Geometry check sheet. Reference: the model listing, model coordinates, mm. Give positions to 0.01 mm unless a question says otherwise; leave off trailing zeros. Write each loop counter-clockwise with the first axis right and the second up, starting at its lowest first coordinate (ties: lowest second). Pieces come first, ordered by that corner, then holes. Notation, with made-up numbers: (65, 21.5) - (123, 21.5) arc R13 ccw to (123, 42.5) - close; hole circle Ø10 at (-3.75, 77). An arc over 180 degrees is marked (long way). Use a Markdown table: item, result.
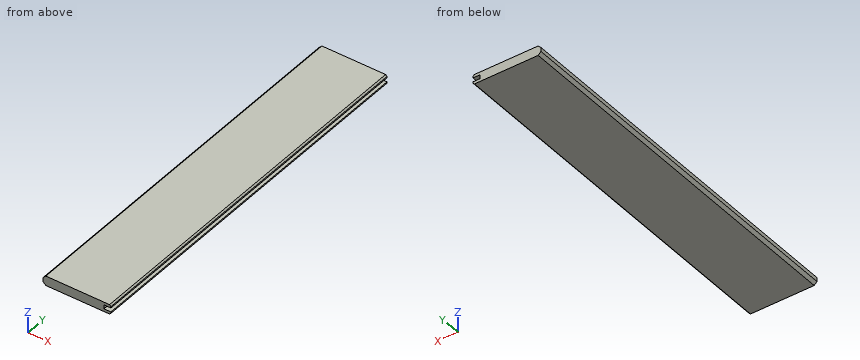
```python
from build123d import *

# Parameters (mm, degrees)
F1_DEPTH = 685.8
F2_SIZE  = 2.54
F3_SIZE  = 5.07999
F4_W     = 25.4
F4_H     = 7.3152
F5_DEPTH = 685.801


# Not quite as in the source:
# - a fillet or chamfer is up to 0.001 mm smaller than in the source, because OpenCascade refuses the exact size


with BuildPart() as f1:
    # F0 (on Front) → F1 (new body)
    with BuildSketch(Plane.XZ):
        Polygon((68.199, 3.6576), (68.199, 8.7376), (-55.499, 8.7376), (-55.499, 3.6576), (-68.199, 3.6576), (-68.199, -3.6576), (-55.499, -3.6576), (-55.499, -8.7376), (68.199, -8.7376), (68.199, -3.6576), (55.499, -3.6576), (55.499, 3.6576), align=None)
    extrude(amount=F1_DEPTH)

    # F2
    f2_edges = [f1.edges().sort_by_distance(p)[0] for p in [
        (68.199, -342.9, 8.7376),
        (68.199, -342.9, -8.7376),
        (-68.199, -342.9, 3.6576),
        (-68.199, -342.9, -3.6576),
    ]]
    chamfer(f2_edges, length=F2_SIZE)

    # F3 (size 5.08 in the source; OpenCascade refuses exactly that, so slightly less here)
    f3_edges = [f1.edges().sort_by_distance(p)[0] for p in [
        (-55.499, -342.9, 8.7376),
        (-55.499, -342.9, -8.7376),
    ]]
    chamfer(f3_edges, length=F3_SIZE)

    # F4 (on face) → F5 (cut, through all)
    with BuildSketch(Plane.XZ.offset(685.8)):
        with Locations((-68.199, 0)):
            Rectangle(F4_W, F4_H)
    extrude(amount=-F5_DEPTH, mode=Mode.SUBTRACT)


solid = f1.part
```
1) Section check A-A on y = -581. Record the boundary of the cut face in (x, z).
Working result:
| item | result |
|---|---|
| outline | (-55.5, -3.66) - (-50.42, -8.74) - (65.66, -8.74) - (68.2, -6.2) - (68.2, -3.66) - (55.5, -3.66) - (55.5, 3.66) - (68.2, 3.66) - (68.2, 6.2) - (65.66, 8.74) - (-50.42, 8.74) - (-55.5, 3.66) - close |
2) Depth check by flat-ended pin: P1, Ø10, axis at x = -16.5, z = -4, coming from the +Y side; P2, Ø1.5, axis at y = -568.5, z = 4.5, coming from the -X side. Enter the tip coordinate at first touch or a pass-through.
Working result:
| item | result |
|---|---|
| P1 | stops at y = 0 |
| P2 | stops at x = -55.41 |
3) Material ranges on L1, parallel to Z at x = 58.5, y = -200.5; L2, parallel to X at y = -44, z = -1; L3, parallel to X at y = -478, z = -6.75, recorded low to high. Write a range as from..to.
Working result:
| item | result |
|---|---|
| L1 | z = -8.74..-3.66, 3.66..8.74 |
| L2 | x = -55.5..55.5 |
| L3 | x = -52.41..67.65 |
4) Section check B-B on z = 0.75. Record the boundary of the cut face in (x, y).
Working result:
| item | result |
|---|---|
| outline | (-55.5, -685.8) - (55.5, -685.8) - (55.5, 0) - (-55.5, 0) - close |
